Read the model definition and answer for the solid it produces. Units are mm, in the model's axes. A direction names the side the tool comes from. Round coordinates to 2 decimals unless told otherwise and drop trailing zeros. Loops run counter-clockwise (first coordinate to the right, second up) from the corner with the lowest first, then second, coordinate; pieces in that order, holes last. Notation, with made-up numbers: (22.5, -9.75) - (56.5, -9.75) arc R24 cw to (56.5, 10.25) - close; hole circle Ø6 at (54.25, 52.5). An arc over 180 degrees is marked (long way). Use CSV: the item, a comma, the result in double quotes. Start each with the question number.
1. A tool of negligible diameter and unlimited length cuts with its end or side. For faces 5 (the flat face through (-1.403, 1.976, -63.768)), 6 (the flat face through (-1.6, 2, -33)), 7 (the flat face through (1.397, 1.976, -3.732)), from which of +Z, -Z, +X, -X, +Y, -Y can it reach the whole face along a straight path? Write none if from no direction.
2. Find section A-A (y = 1.95). Give the vertices of the cut face in (x, z).
3. Determine the mould class of faces 1 (the flat face through (-1.397, 1.976, -1.267)), 2 (the flat face through (0, 2, 0)), 3 (the flat face through (0, 2, -65)), 4 (the flat face through (1.403, 1.976, -1.233)) for opening direction Z: +Z half, -Z half, draft (parallel to the pull), parting line (faces both ways), or undercut.
4. Consider line 1 along X through (y, z) = (2.4, -62); line 2 along X through (y, z) = (3.45, -4). Determine where each line is inside the solid, lowest interval first.
from build123d import *

# Parameters (mm, degrees)
BOSS_EXTRUDE1_DEPTH = 4
CHAMFER1_SIZE       = 0.25


with BuildPart() as part:
    # Sketch1 → Boss-Extrude1 (new body)
    with BuildSketch(Plane(origin=(0, 0, 0), x_dir=(1, 0, 0), z_dir=(0, 1, 0))):
        Polygon((-1.6, 0), (1.6, 0), (1.2, 2.5), (1.6, 5), (1.6, 60), (1.2, 62.5), (1.6, 65), (-1.6, 65), (-1.2, 62.5), (-1.6, 60), (-1.6, 5), (-1.2, 2.5), align=None)
    extrude(amount=BOSS_EXTRUDE1_DEPTH)

    # Chamfer1
    chamfer1_edges = [part.edges().sort_by_distance(p)[0] for p in [
        (-1.4, 0, -3.75),
        (-1.6, 0, -32.5),
        (1.4, 4, -1.25),
        (-1.4, 0, -61.25),
        (-1.4, 0, -63.75),
        (0, 0, -65),
        (1.4, 0, -63.75),
        (1.4, 0, -61.25),
        (1.6, 0, -32.5),
        (1.4, 0, -3.75),
        (1.4, 0, -1.25),
        (0, 0, 0),
        (-1.4, 0, -1.25),
        (1.4, 4, -3.75),
        (1.6, 4, -32.5),
        (1.4, 4, -61.25),
        (1.4, 4, -63.75),
        (0, 4, -65),
        (-1.4, 4, -63.75),
        (-1.4, 4, -61.25),
        (-1.6, 4, -32.5),
        (-1.4, 4, -3.75),
        (-1.4, 4, -1.25),
        (0, 4, 0),
    ]]
    chamfer(chamfer1_edges, length=CHAMFER1_SIZE)


solid = part.part
Filled sheet:
1,face 5,"-X, +Y, -Y"
1,face 6,"+Z, -Z, -X, +Y, -Y"
1,face 7,"+X, +Y, -Y"
2,outline,"(-1.6, -65) - (1.6, -65) - (1.2, -62.5) - (1.6, -60) - (1.6, -5) - (1.2, -2.5) - (1.6, 0) - (-1.6, 0) - (-1.2, -2.5) - (-1.6, -5) - (-1.6, -60) - (-1.2, -62.5) - close"
3,face 1,"undercut"
3,face 2,"+Z half"
3,face 3,"-Z half"
3,face 4,"undercut"
4,line 1,"x = -1.28 to 1.28"
4,line 2,"x = -1.44 to 1.44"
